Geometry check sheet. Reference: the model listing, model coordinates, mm. A direction names the side the tool comes from. Round coordinates to 2 decimals unless told otherwise and drop trailing zeros. Write each loop counter-clockwise with the first axis right and the second up, starting at its lowest first coordinate (ties: lowest second). Pieces come first, ordered by that corner, then holes. Notation, with made-up numbers: (68, 51) - (80, 51) arc R16 cw to (80, 68) - close; hole circle Ø2 at (13.5, 85.25). An arc over 180 degrees is marked (long way). Return JSON: item names as keys, results as strings. Group by question number.
from build123d import *

# Parameters (mm, degrees)
SKETCH1_W           = 6.18
SKETCH1_H           = 11.5
SKETCH1_W_2         = 3.18
SKETCH1_H_2         = 8.5
BOSS_EXTRUDE1_DEPTH = 4.88
SKETCH2_W           = 6.18
SKETCH2_H           = 11.5
BOSS_EXTRUDE2_DEPTH = 1
SKETCH3_W           = 6.18
SKETCH3_H           = 4.16
BOSS_EXTRUDE3_DEPTH = 10
SKETCH4_R           = 1.47
CUT_EXTRUDE1_DEPTH  = 17.587718348


with BuildPart() as part:
    # Sketch1 → Boss-Extrude1 (new body)
    with BuildSketch(Plane.XY):
        with Locations((1.59, 4.25)):
            Rectangle(SKETCH1_W, SKETCH1_H)
        with Locations((1.59, 4.25)):
            Rectangle(SKETCH1_W_2, SKETCH1_H_2, mode=Mode.SUBTRACT)
    extrude(amount=BOSS_EXTRUDE1_DEPTH)

    # Sketch2 → Boss-Extrude2 (add)
    with BuildSketch(Plane(origin=(0, 0, 0), x_dir=(-1, 0, 0), z_dir=(0, 0, -1))):
        with Locations((-1.59, 4.25)):
            Rectangle(SKETCH2_W, SKETCH2_H)
    extrude(amount=BOSS_EXTRUDE2_DEPTH)

    # Sketch3 → Boss-Extrude3 (add)
    with BuildSketch(Plane(origin=(0, 0, -1), x_dir=(-1, 0, 0), z_dir=(0, 0, -1))):
        with Locations((-1.59, 7.92)):
            Rectangle(SKETCH3_W, SKETCH3_H)
        with Locations((-1.59, 0.58)):
            Rectangle(SKETCH3_W, SKETCH3_H)
    extrude(amount=BOSS_EXTRUDE3_DEPTH)

    # Sketch4 → Cut-Extrude1 (cut, through all)
    with BuildSketch(Plane(origin=(0, 10, 0), x_dir=(1, 0, 0), z_dir=(0, 1, 0))):
        with Locations(Location((1.59, 3.5, 0), (0, 0, 270))):
            Circle(SKETCH4_R)
        with Locations(Location((1.59, 8.5, 0), (0, 0, 270))):
            Circle(SKETCH4_R)
    extrude(amount=-CUT_EXTRUDE1_DEPTH, mode=Mode.SUBTRACT)


solid = part.part
1. Mould release check, pull along Z, two halves, no side actions. Record for faces 1 (the face through (1.65, 7.95, -4.97)), 2 (the face through (1.03, 0.61, -7.14)), 3 (the face through (2, -1.5, -1)), 4 (the face through (2, 4, -1)): pulls with the +Z half, pulls with the -Z half, needs draft (parallel to the pull), parting line crosses it, or undercut.
2. Tool access check on faces 5 (the face through (3.18, 4, 2)), 6 (the face through (1.65, 0.61, -4.97)), 7 (the face through (2, 5.84, -6)). Record the directions out of +Z, -Z, +X, -X, +Y, -Y that give a thin tool (end or side, any length) a straight path to the whole face; none if there is none.
3. Section check D-D (y = 3). Enter the section's corners in (x, z).
4. Section check C-C (z = -3.5). Enter the section's corners in (x, y), and give its area (3 significant figures).
5. Depth check by flat-ended pin: pin 1 Ø2.5 at (x, z) = (1.59, -3.5) entering from +Y; pin 2 Ø2 at (x, y) = (0, 5.5) entering from -Z; pin 3 Ø1.6 at (x, y) = (2, 4) entering from -Z. Enter the tip coordinate at first touch or a pass-through.
6. Section check A-A (x = 1.59). Enter the section's corners in (y, z).
7. Section check B-B (y = 9). Enter the section's corners in (x, z), and give its area (3 significant figures).
8. Material ranges on line 1 along Y through (x, z) = (0.75, -6); line 2 along Y through (x, z) = (2.75, 3.25); line 3 along X through (y, z) = (9.1, -3.5), recorded low to high.
Result sheet:
{
 "1": {"face 1": "undercut", "face 2": "undercut", "face 3": "needs draft", "face 4": "pulls with the -Z half"},
 "2": {"face 5": "+Z", "face 6": "+Y, -Y", "face 7": "-Z, +X, -X"},
 "3": {"outline": "(-1.5, -1) - (4.68, -1) - (4.68, 4.88) - (3.18, 4.88) - (3.18, 0) - (0, 0) - (0, 4.88) - (-1.5, 4.88) - close"},
 "4": {"outline": "(-1.5, -1.5) - (0.12, -1.5) - (0.12, 2.66) - (-1.5, 2.66) - close; (-1.5, 5.84) - (0.12, 5.84) - (0.12, 10) - (-1.5, 10) - close; (3.06, -1.5) - (4.68, -1.5) - (4.68, 2.66) - (3.06, 2.66) - close; (3.06, 5.84) - (4.68, 5.84) - (4.68, 10) - (3.06, 10) - close", "area": "27.0 mm²"},
 "5": {"pin 1": "passes through", "pin 2": "stops at z = -11", "pin 3": "stops at z = -1"},
 "6": {"outline": "(-1.5, -11) - (2.66, -11) - (2.66, -9.97) - (-1.5, -9.97) - close; (-1.5, -7.03) - (2.66, -7.03) - (2.66, -4.97) - (-1.5, -4.97) - close; (-1.5, -2.03) - (2.66, -2.03) - (2.66, -1) - (5.84, -1) - (5.84, -2.03) - (10, -2.03) - (10, 4.88) - (8.5, 4.88) - (8.5, 0) - (0, 0) - (0, 4.88) - (-1.5, 4.88) - close; (5.84, -11) - (10, -11) - (10, -9.97) - (5.84, -9.97) - close; (5.84, -7.03) - (10, -7.03) - (10, -4.97) - (5.84, -4.97) - close"},
 "7": {"outline": "(-1.5, -11) - (4.68, -11) - (4.68, 4.88) - (-1.5, 4.88) - close; hole circle Ø2.94 at (1.59, -8.5); hole circle Ø2.94 at (1.59, -3.5)", "area": "84.6 mm²"},
 "8": {"line 1": "y = -1.5 to 2.66, 5.84 to 10", "line 2": "y = -1.5 to 0, 8.5 to 10", "line 3": "x = -1.5 to 0.12, 3.06 to 4.68"}
}
